CAD build for the part. Positions are in the model's coordinates, mm. A direction names the side the tool comes from. Coordinates: 2 decimals unless noted, no trailing zeros. Loops run counter-clockwise (first coordinate to the right, second up) from the corner with the lowest first, then second, coordinate; pieces in that order, holes last. Notation, with made-up numbers: (37.5, 8) -> (66.5, 8) arc R13 cw to (66.5, 33) -> close; hole circle Ø2 at (82, -28.75). An arc over 180 degrees is marked (long way). Answer as a JSON object with one key per item and string values. Group by question number.
from build123d import *

# Parameters (mm, degrees)
F1_W          = 10
F1_H          = 6
F3_DEPTH      = 100
F3_DEPTH_BACK = 100
F5_DEPTH      = 100
F6_R          = 5


with BuildPart() as f2:
    # F0 (on Top) → F2 (revolve)
    with BuildSketch(Plane.XY):
        Polygon((0, -50), (0, -15), (-50, -15), (-50, -30), (-20, -30), (-20, -50), align=None)
    revolve(axis=Axis((-24.532024, 0, 0), (-1, 0, 0)))

    # F1 (on Front) → F3 (cut, two sides)
    with BuildSketch(Plane.XZ) as f3_sk:
        with Locations((-5, 3)):
            Rectangle(F1_W, F1_H)
        with Locations((-5, -3)):
            Rectangle(F1_W, F1_H)
    extrude(amount=F3_DEPTH, mode=Mode.SUBTRACT)
    extrude(f3_sk.sketch, amount=-F3_DEPTH_BACK, mode=Mode.SUBTRACT)

    # F4 (on Right) → F5 (cut)
    with BuildSketch(Plane.YZ):
        with BuildLine():
            ThreePointArc((-15, 0), (-14.924042, 1.507634), (-14.696938, 3))
            Line((-14.696938, 3), (-17.696938, 3))
            Line((-17.696938, 3), (-17.696938, 0))
            Line((-17.696938, 0), (-15, 0))
        make_face()
        with BuildLine():
            Line((-17.696938, -3), (-14.696938, -3))
            ThreePointArc((-14.696938, -3), (-14.924042, -1.507634), (-15, 0))
            Line((-15, 0), (-17.696938, 0))
            Line((-17.696938, 0), (-17.696938, -3))
        make_face()
    extrude(amount=-F5_DEPTH, mode=Mode.SUBTRACT)

    # F6
    f6_edges = [f2.edges().sort_by_distance(p)[0] for p in [
        (-20, 30, 0),
    ]]
    fillet(f6_edges, radius=F6_R)


solid = f2.part
Item 1: Band-saw the part on A-A, the plane y = 0. List the corners of the cut face in (x, z).
Item 2: Band-saw the part on C-C, the plane x = -3.5. List the corners of the cut face in (y, z), and give its area (3 significant figures).
Item 3: Pull direction Z, two halves, no side cores. Call faces 1 (the flat face through (0, 1, -28)), 2 (the cylindrical face through (-9.86, -47.69, 15.02)), 3 (the flat face through (-5, -31, 6)): +Z half, -Z half, draft (parallel to the pull), parting line (faces both ways), or undercut.
Item 4: Drill centre lines: L1, parallel to Z at x = -37.5, y = 0; L2, parallel to Y at x = -17.5, z = 0; L3, parallel to Z at x = -16, y = 0. Where is each one in solid material? Low to high.
Item 5: Band-saw the part on D-D, the plane x = -14. List the corners of the cut face in (y, z), and give its area (3 significant figures).
Item 6: 3-axis set-ups, long thin cutter, end or side, ignore diameter. For faces 4 (the flat face through (-50, 6, 14)), 5 (the flat face through (-20, -34, -10)), 6 (the flat face through (-10, 32, 0)), 7 (the flat face through (-30, -17.697, 0)): which of +Z, -Z, +X, -X, +Y, -Y reach the whole face in a straight line?
Item 7: Band-saw the part on B-B, the plane z = 0. List the corners of the cut face in (x, y).
Item 8: Flat gauge pins, fed straight in: P1, Ø0.9, axis at x = -22, y = -15.5, coming from the +Z side; P2, Ø5, axis at x = -6.5, y = -33, coming from the +Z side; P3, Ø6.5, axis at x = -27.5, z = 1, coming from the +Y side. Where does each tip first touch, or does it go through?
Reply:
{
 "1": {"outline": "(-50, -30) -> (-25, -30) arc R5 cw to (-20, -35) -> (-20, -50) -> (0, -50) -> (0, -15) -> (-50, -15) -> close; (-50, 15) -> (0, 15) -> (0, 50) -> (-20, 50) -> (-20, 35) arc R5 cw to (-25, 30) -> (-50, 30) -> close"},
 "2": {"outline": "(-49.64, -6) arc R50 ccw to (49.64, -6) -> (13.75, -6) arc R15 cw to (-13.75, -6) -> close; (-49.64, 6) -> (-13.75, 6) arc R15 cw to (13.75, 6) -> (49.64, 6) arc R50 ccw to start", "area": "6,300 mm²"},
 "3": {"face 1": "draft", "face 2": "parting line", "face 3": "undercut"},
 "4": {"L1": "-30 to -15, 15 to 30", "L2": "-50 to -17.7, 15 to 50", "L3": "-50 to -15, 15 to 50"},
 "5": {"outline": "circle Ø100 at (0, 0); hole (-17.7, -3) -> (-14.7, -3) arc R15 ccw (long way) to (-14.7, 3) -> (-17.7, 3) -> close", "area": "7,130 mm²"},
 "6": {"face 4": "+Z, -Z, -X, +Y, -Y", "face 5": "-X", "face 6": "+X, +Y, -Y", "face 7": "+X, -X"},
 "7": {"outline": "(-50, -30) -> (-25, -30) arc R5 cw to (-20, -35) -> (-20, -50) -> (-10, -50) -> (-10, -17.7) -> (-50, -17.7) -> close; (-50, 15) -> (-10, 15) -> (-10, 50) -> (-20, 50) -> (-20, 35) arc R5 cw to (-25, 30) -> (-50, 30) -> close"},
 "8": {"P1": "z = 27.35", "P2": "z = 39.62", "P3": "y = 30.05"}
}
